Read the model definition and answer for the solid it produces. Units are mm, in the model's axes. Face numbers are marked on the shaded views. A direction names the side the tool comes from. Give positions to 0.01 mm unless a question says otherwise; leave off trailing zeros. Write each loop counter-clockwise with the first axis right and the second up, starting at its lowest first coordinate (ties: lowest second). Pieces come first, ordered by that corner, then holes. Notation, with made-up numbers: M -24,70 L 35,70 A27 cw 35,99 Z; hole C 17.25,-39 d11. An arc over 180 degrees is marked long. Put each result on its own line as item: value.
from build123d import *

# Parameters (mm, degrees)
SKETCH1_W           = 12.192
SKETCH1_H           = 4.4958
BOSS_EXTRUDE1_DEPTH = 12.446
BOSS_EXTRUDE2_DEPTH = 3.8862
FILLET1_R           = 5.08
FILLET2_R           = 1.27
SKETCH3_R           = 0.705537126
CUT_EXTRUDE1_DEPTH  = 0.254


# Read off the part's stored shape, not the designer's step: Mirror1
with BuildPart() as part:
    # Sketch1 → Boss-Extrude1 (new body)
    with BuildSketch(Plane(origin=(0, 0, 0), x_dir=(1, 0, 0), z_dir=(0, 1, 0))):
        Rectangle(SKETCH1_W, SKETCH1_H)
    extrude(amount=BOSS_EXTRUDE1_DEPTH)

    # Sketch2 → Boss-Extrude2 (add, symmetric)
    with BuildSketch(Plane.XY):
        with BuildLine():
            Line((0, 0), (-8.4074, 0))
            ThreePointArc((-8.4074, 0), (-8.750605066, -11.506432361), (-9.779, -22.971953685))
            ThreePointArc((-9.779, -22.971953685), (-4.945799179, -24.086008668), (0, -24.4602))
            Line((0, -24.4602), (0, 0))
        make_face()
    extrude(amount=BOSS_EXTRUDE2_DEPTH, both=True)

    # Fillet1
    fillet1_edges = [part.edges().sort_by_distance(p)[0] for p in [
        (-4.945799179, -24.086008668, 3.8862),
    ]]
    fillet(fillet1_edges, radius=FILLET1_R)

    # Fillet2
    fillet2_edges = [part.edges().sort_by_distance(p)[0] for p in [
        (-4.945799179, -24.086008668, -3.8862),
        (-8.61315874, -8.910874841, 3.8862),
        (-9.779, -22.971953685, -2.54),
        (-9.601797377, -21.441669836, 2.422651407),
    ]]
    fillet(fillet2_edges, radius=FILLET2_R)

    # Mirror1: part across plane


with BuildPart() as part_1:
    add(part.part)
    add(part.part.mirror(Plane(origin=(0, 0, 0), x_dir=(0, 0, 1), z_dir=(1, 0, 0))))

    # Sketch3 → Cut-Extrude1 (cut)
    with BuildSketch(Plane.XY.offset(3.8862)):
        with Locations((-3.72090503, -5.794071086)):
            Circle(SKETCH3_R)
    extrude(amount=-CUT_EXTRUDE1_DEPTH, mode=Mode.SUBTRACT)


solid = part_1.part
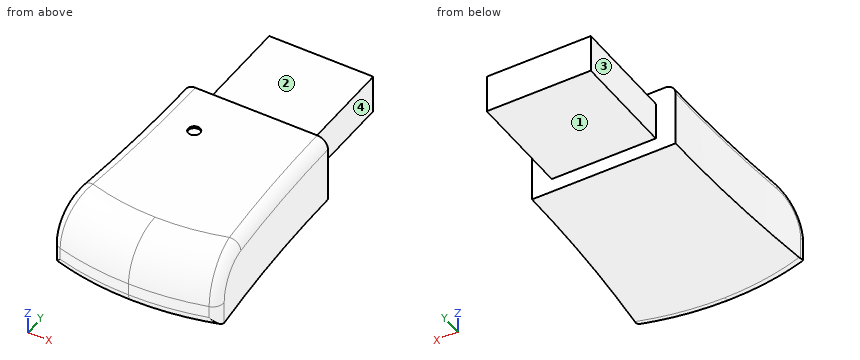
(1) Which of the six approach directions +Z, -Z, +X, -X, +Y, -Y give full straight-line access (tool end or side, diameter ignored) to the marked faces 1, 2, 3 and 4?
Result:
face 1: -Z, +X, -X, +Y
face 2: +Z, +X, -X, +Y
face 3: +Z, -Z, -X, +Y
face 4: +Z, -Z, +X, +Y
(2) Given pin 1 Ø2 at (y, z) = (8, 1) entering from -X; pin 2 Ø1 at (y, z) = (-20, 3) entering from +X; pin 3 Ø3 at (y, z) = (-18, -2) entering from -X, each flat-ended and moving along its own axis, determine where each tip first touches the part or whether it passes through.
Result:
pin 1: stops at x = -6.1
pin 2: stops at x = 9.4
pin 3: stops at x = -9.39
(3) Section A-A on y = 6.5 is taken. Determine the outline of the cut face in (x, z), and give its area (3 significant figures).
Result:
outline: M -6.1,-2.25 L 6.1,-2.25 L 6.1,2.25 L -6.1,2.25 Z
area: 54.8 mm²
(4) Straight lines are drawn through the part: line 1 along X through (y, z) = (6, -0.25); line 2 along X through (y, z) = (-1, -0.5); line 3 along Y through (x, z) = (-4.75, -0.5). For each, find the intervals that lie inside material, in ascending order. Write a range as from..to.
Result:
line 1: x = -6.1..6.1
line 2: x = -8.41..8.41
line 3: y = -24.07..12.45
